The figure shows three views and two pictorial views of one solid part (mm, origin at its lowest corner). Answer the questions. Round coordinates to 2 decimals unless told otherwise and drop trailing zeros. Write each loop counter-clockwise with the first axis right and the second up, starting at its lowest first coordinate (ties: lowest second). Pieces come first, ordered by that corner, then holes. Notation, with made-up numbers: M 25.5,21 L 56.5,21 A16 ccw 56.5,46 Z; hole C 83,-6.5 d4. An arc over 180 degrees is marked long. Answer in a Markdown table with one row per item.
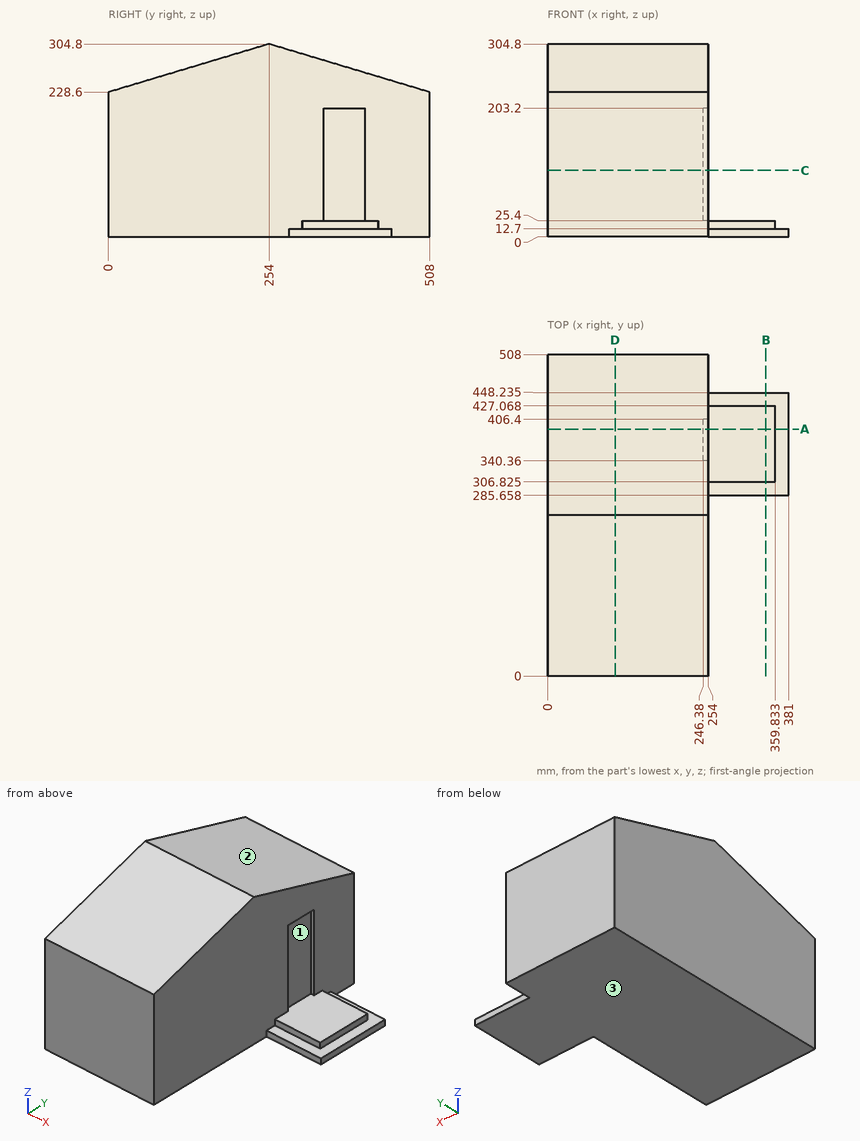
1. The part is cut by section D-D (x = 106.5). Determine the outline of the cut face in (y, z), plus the area to 3 significant figures.
Calculated:
| item | result |
|---|---|
| outline | M 0,0 L 508,0 L 508,228.6 L 254,304.8 L 0,228.6 Z |
| area | 135,000 mm² |
2. Consider line 1 along X through (y, z) = (481, 131); line 2 along Z through (x, y) = (339, 359); line 3 along X through (y, z) = (345.5, 79). Determine where each line is inside the solid, lowest interval first. Write a range as from..to.
Calculated:
| item | result |
|---|---|
| line 1 | x = 0..254 |
| line 2 | z = 0..25.4 |
| line 3 | x = 0..246.38 |
3. The part is cut by section C-C (z = 105). Determine the outline of the cut face in (x, y).
Calculated:
| item | result |
|---|---|
| outline | M 0,0 L 254,0 L 254,340.36 L 246.38,340.36 L 246.38,406.4 L 254,406.4 L 254,508 L 0,508 Z |
4. Given pin 1 (5 mm diameter, centred on y = 333.5, z = 59, fed in from -X); pin 2 (14 mm diameter, centred on x = 294, z = 5, fed in from +Y) (1 decimal); pin 3 (14 mm diameter, centred on y = 351, z = 20.5, fed in from +X); pin 4 (6.5 mm diameter, centred on x = 327, z = 17, fed in from -Y) (1 decimal), each flat-ended and moving along its own axis, determine where each tip first touches the part or whether it passes through.
Calculated:
| item | result |
|---|---|
| pin 1 | stops at x = 0 |
| pin 2 | stops at y = 448.2 |
| pin 3 | stops at x = 359.83 |
| pin 4 | stops at y = 306.8 |
5. The part is cut by section B-B (x = 345). Determine the outline of the cut face in (y, z) (1 decimal), plus the area to 3 significant figures.
Calculated:
| item | result |
|---|---|
| outline | M 285.7,0 L 448.2,0 L 448.2,12.7 L 427.1,12.7 L 427.1,25.4 L 306.8,25.4 L 306.8,12.7 L 285.7,12.7 Z |
| area | 3,590 mm² |
6. The part is cut by section A-A (y = 390.5). Determine the outline of the cut face in (x, z).
Calculated:
| item | result |
|---|---|
| outline | M 0,0 L 381,0 L 381,12.7 L 359.83,12.7 L 359.83,25.4 L 246.38,25.4 L 246.38,203.2 L 254,203.2 L 254,263.85 L 0,263.85 Z |
7. Determine the mould class of the marked faces 1, 2 and 3 for opening direction Y: released by +Y, released by -Y, zero draft, split by the parting line, or undercut.
Calculated:
| item | result |
|---|---|
| face 1 | undercut |
| face 2 | released by +Y |
| face 3 | zero draft |
